The model under review builds one solid part; all positions refer to its coordinate system, in mm. Face numbers are marked on the shaded views. A direction names the side the tool comes from. Coordinates: 2 decimals unless noted, no trailing zeros. Write each loop counter-clockwise with the first axis right and the second up, starting at its lowest first coordinate (ties: lowest second). Pieces come first, ordered by that corner, then holes.
1) Machinability: for the marked faces 1, 2 and 3, which of the approach directions +Z, -Z, +X, -X, +Y, -Y give a long, thin tool a straight path to every point of the face, cutting with its end or side? Answer none if there is none.
2) Add section B-B, the plane y = 0. State the section outline as (x, z) points (3 decimals), then the cut area to 3 significant figures.
3) Add section A-A, the plane x = 0. State the section outline as (y, z) points (3 decimals), then the cut area to 3 significant figures.
4) Mouldability with a two-part tool opening along Z and no side actions: class the marked faces 4, 5, 6 and 7 as released by +Z, released by -Z, zero draft, split by the parting line, or undercut.
5) Add section C-C, the plane z = 5. State the section outline as (x, y) points (3 decimals).
6) For P1, Ø4, axis at y = -4.5, z = -0.5, coming from the +X side; P2, Ø2, axis at x = -3.5, z = 6, coming from the -Y side; P3, Ø5, axis at y = 0, z = 5, coming from the -X side, all flat-tipped, find the tip position at first contact; note any pin that passes through.
7) For line 1 (Y direction, x = 0, z = -1) (3 decimals); line 2 (Z direction, x = 2, y = 5.5); line 3 (Y direction, x = -4.1, z = 5), list the stretches that pass through material, from the lowest coordinate up.
8) Add section D-D, the plane z = -1. State the section outline as (x, y) points (3 decimals), then the cut area to 3 significant figures.
Autodesk Inventor part; units mm, degrees
ref_plane "XZ Plane" through (0, 0, 0) normal (0, 1, 0) x (-1, 0, 0)
ref_plane "XY Plane" through (0, 0, 0) normal (0, 0, 1) x (1, 0, 0)
sketch "Sketch1" plane through (0, 0, 0) normal (0, 0, 1) x (1, 0, 0)
  circle A0 centre (0, 0) radius 5
  circle A1 centre (0, 0) radius 3.175
  dimension "d0" = 10
  dimension "d1" = 6.35
extrude "Extrusion1" add sketch "Sketch1" along normal blind 10
sketch "Sketch2" plane through (0, 0, 10) normal (0, 0, 1) x (1, 0, 0)
  circle A0 centre (0, 0) radius 6.5
  circle A1 centre (0, 0) radius 3.175
  dimension "d4" = 13
sketch "Sketch4" plane through (0, 0, 0) normal (0, 0, -1) x (-1, 0, 0)
  circle A0 centre (0, 0) radius 6.5
  circle A1 centre (0, 0) radius 3.175
  dimension "d8" = 13
extrude "Extrusion4" add sketch "Sketch2" along normal blind 2
extrude "Extrusion5" add sketch "Sketch4" along normal blind 2
ref_plane "Work Plane1" through (5, 0, 0) normal (1, 0, 0) x (0, 1, 0)
sketch "Sketch5" plane through (5, 0, 0) normal (1, 0, 0) x (0, 1, 0)
  line L0 (6.5, 0) -> (-6.5, 0)
  line L1 (-6.5, 10) -> (6.5, 10)
  line L2 (0, 0) -> (0, 10)
  point P0 (0, 5)
hole "Hole1" at (5, 0, 5) direction (-1, 0, 0) diameter 3 end through all counterbore diameter 4 counterbore depth 3
ref_plane "Work Plane2" through (-5, 0, 0) normal (1, 0, 0) x (0, 1, 0)
sketch "Sketch6" plane through (-5, 0, 0) normal (1, 0, 0) x (0, 1, 0)
  line L0 (0, 3.5) -> (0, 3.5)
  point P0 (0, 0)
  point P1 (1.5, 5)
equation "\"d13\" = lip"
equation "\"d15\" = lip"
properties part number "firstSpindle"
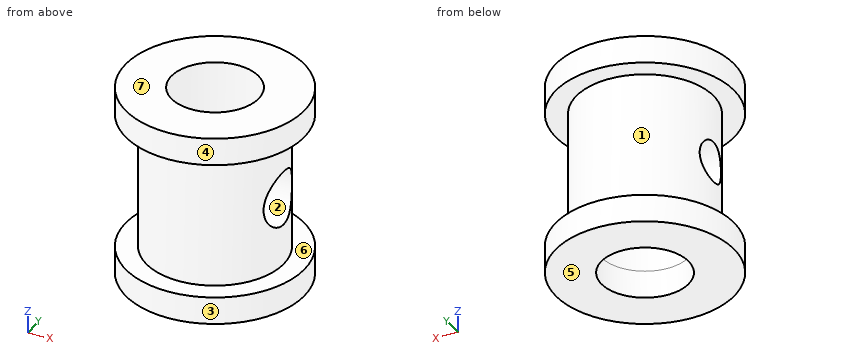
Geometry results:
1. face 1: none
1. face 2: +X
1. face 3: +Z, -Z
2. outline: (-6.5, -2) - (-3.175, -2) - (-3.175, 3.5) - (-5, 3.5) - (-5, 0) - (-6.5, 0) - close; (-6.5, 10) - (-5, 10) - (-5, 6.5) - (-3.175, 6.5) - (-3.175, 12) - (-6.5, 12) - close; (3.175, -2) - (6.5, -2) - (6.5, 0) - (5, 0) - (5, 3) - (3.175, 3) - close; (3.175, 7) - (5, 7) - (5, 10) - (6.5, 10) - (6.5, 12) - (3.175, 12) - close
2. area: 50.3 mm2
3. outline: (-6.5, -2) - (-3.175, -2) - (-3.175, 12) - (-6.5, 12) - (-6.5, 10) - (-5, 10) - (-5, 0) - (-6.5, 0) - close; (3.175, -2) - (6.5, -2) - (6.5, 0) - (5, 0) - (5, 10) - (6.5, 10) - (6.5, 12) - (3.175, 12) - close
3. area: 63.1 mm2
4. face 4: zero draft
4. face 5: released by -Z
4. face 6: undercut
4. face 7: released by +Z
5. outline: (-4.77, -1.5) arc R5 ccw to (4.583, -2) - (2.466, -2) arc R3.175 cw to (-2.798, -1.5) - close; (-4.77, 1.5) - (-2.798, 1.5) arc R3.175 cw to (2.466, 2) - (4.583, 2) arc R5 ccw to start
6. P1: stops at x = 6
6. P2: stops at y = -4.33
6. P3: stops at x = -5
7. line 1: y = -6.5 to -3.175, 3.175 to 6.5
7. line 2: z = -2 to 0, 10 to 12
7. line 3: y = -2.86 to -1.5, 1.5 to 2.86
8. outline: circle Ø13 at (0, 0); hole circle Ø6.35 at (0, 0)
8. area: 101 mm2
